```python
from build123d import *

# Parameters (mm, degrees)
F1_DEPTH = 63.5
F0_W     = 25.4
F0_H     = 19.05
F2_DEPTH = 25.4
F3_DEPTH = 15.875
F5_R     = 6.35


with BuildPart() as f1:
    # F0 (on Front) → F1 (new body, symmetric)
    with BuildSketch(Plane.XZ):
        Polygon((-41.275, 9.525), (-41.275, -9.525), (41.275, -9.525), (41.275, 9.525), (22.225, 9.525), align=None)
    extrude(amount=F1_DEPTH, both=True)

    # F0 (on Front) → F2 (join, symmetric)
    with BuildSketch(Plane.XZ):
        Polygon((60.325, 66.675), (60.325, 61.9252), (85.725, 61.9252), (85.725, 42.8752), (60.325, 42.8752), (60.325, 34.925), (111.125, 34.925), (111.125, 66.675), align=None)
        with BuildLine():
            Line((22.225, 9.525), (41.275, 9.525))
            Line((41.275, 9.525), (41.275, 27.0002))
            ThreePointArc((41.275, 27.0002), (45.92468, 38.22552), (57.15, 42.8752))
            Line((57.15, 42.8752), (60.325, 42.8752))
            Line((60.325, 42.8752), (60.325, 61.9252))
            Line((60.325, 61.9252), (57.15, 61.9252))
            ThreePointArc((57.15, 61.9252), (32.454296, 51.695904), (22.225, 27.0002))
            Line((22.225, 27.0002), (22.225, 9.525))
        make_face()
        with Locations((73.025, 52.4002)):
            Rectangle(F0_W, F0_H)
    extrude(amount=F2_DEPTH, both=True)

    # F0 (on Front) → F3 (join)
    with BuildSketch(Plane.XZ):
        with BuildLine():
            add(Edge.make_bspline(
                [(-41.275, 9.525), (-27.823856, 40.664345), (5.336885, 65.223247), (57.15, 61.9252)],
                knots=[0, 0, 0, 0, 111.504536, 111.504536, 111.504536, 111.504536], degree=3))
            Line((-41.275, 9.525), (22.225, 9.525))
            Line((22.225, 9.525), (22.225, 27.0002))
            ThreePointArc((22.225, 27.0002), (32.454296, 51.695904), (57.15, 61.9252))
        make_face()
    extrude(amount=F3_DEPTH)

    # F0 (on Front) → F4 (revolve)
    with BuildSketch(Plane.XZ):
        Polygon((60.325, 66.675), (60.325, 61.9252), (85.725, 61.9252), (85.725, 42.8752), (60.325, 42.8752), (60.325, 34.925), (111.125, 34.925), (111.125, 66.675), align=None)
    revolve(axis=Axis((111.125, 0, 50.8), (0, 0, 1)))

    # F5
    f5_edges = [f1.edges().sort_by_distance(p)[0] for p in [
        (-41.275, -63.5, 0),
        (41.275, -63.5, 0),
        (41.275, 63.5, 0),
        (-41.275, 63.5, 0),
    ]]
    fillet(f5_edges, radius=F5_R)


solid = f1.part
```
Can you work these out from the model? Positions are in its coordinate system, mm. A direction names the side the tool comes from. Coordinates: 2 decimals unless noted, no trailing zeros. Loops run counter-clockwise (first coordinate to the right, second up) from the corner with the lowest first, then second, coordinate; pieces in that order, holes last.
1) Imagine slicing it at A-A on y = 47. List the corners of the cut face in (x, z) for me (3 decimals), plus the area to 3 significant figures.
2) I need wall thicknesses on probe 1 along Z at (x, y) = (141, -13.5) (3 decimals); probe 2 along Z at (x, y) = (79, 10) (3 decimals); probe 3 along X at (y, z) = (-9, -2) (3 decimals). Which ranges of each line are inside material? Lowest first, please.
3) Which directions (+Z, -Z, +X, -X, +Y, -Y) give clear straight access to the entire face, cutting with the end or side of a thin tool? Please do faces 1 (the flat face through (-2, -15.875, 32)), 2 (the flat face through (135, 11, 42.875)), 3 (the cylindrical face through (45.8, -0.4, 38.1)).
4) Thinking about a two-plate mould opening in Z: for faces 4 (the cylindrical face through (32.73, 12.52, 51.97)), 5 (the flat face through (56, -25.4, 45)), 6 (the cylindrical face through (39.365, 61.689, 0.133)), 7 (the flat face through (136, 11, 61.925)), which applies, pulls with the +Z half, pulls with the -Z half, needs draft (parallel to the pull), parting line crosses it, or undercut?
5) For pin 1 (2.5 mm diameter, centred on x = 58.5, y = 5, fed in from +Z); pin 2 (1 mm diameter, centred on x = 69, z = 33.5, fed in from +Y); pin 3 (2.5 mm diameter, centred on y = -11, z = 38, fed in from -X); pin 4 (10 mm diameter, centred on x = 104.5, y = -28.5, fed in from -Z) (3 decimals), each with a flat end and sliding along its axis, tell me the tip position at first contact or that it passes through.
6) Imagine slicing it at B-B on z = 7. List the corners of the cut face in (x, y) for me (3 decimals).
7) Imagine slicing it at C-C on y = 5.5. List the corners of the cut face in (x, z) for me (3 decimals), plus the area to 3 significant figures.
8) Imagine slicing it at D-D on y = 30. List the corners of the cut face in (x, z) for me (3 decimals).
Completed:
1. outline: (-41.275, -9.525) - (41.275, -9.525) - (41.275, 9.525) - (-41.275, 9.525) - close; (91.847, 34.925) - (130.403, 34.925) - (130.403, 42.875) - (91.847, 42.875) - close; (91.847, 61.925) - (130.403, 61.925) - (130.403, 66.675) - (91.847, 66.675) - close
1. area: 2,060 mm2
2. probe 1: z = 34.925 to 42.875, 61.925 to 66.675
2. probe 2: z = 34.925 to 66.675
2. probe 3: x = -41.275 to 41.275
3. face 1: +Z, -X, -Y
3. face 2: +X
3. face 3: -Z, +Y, -Y
4. face 4: pulls with the +Z half
4. face 5: undercut
4. face 6: needs draft
4. face 7: undercut
5. pin 1: stops at z = 61.93
5. pin 2: passes through
5. pin 3: stops at x = -22.29
5. pin 4: stops at z = 34.925
6. outline: (-41.275, -57.15) arc R6.35 ccw to (-34.925, -63.5) - (34.925, -63.5) arc R6.35 ccw to (41.275, -57.15) - (41.275, 57.15) arc R6.35 ccw to (34.925, 63.5) - (-34.925, 63.5) arc R6.35 ccw to (-41.275, 57.15) - close
7. outline: (-41.275, -9.525) - (41.275, -9.525) - (41.275, 27) arc R15.875 cw to (57.15, 42.875) - (60.325, 42.875) - (60.325, 34.925) - (161.626, 34.925) - (161.626, 42.875) - (135.922, 42.875) - (135.922, 61.925) - (161.626, 61.925) - (161.626, 66.675) - (60.325, 66.675) - (60.325, 61.925) - (57.15, 61.925) arc R34.925 ccw to (22.225, 27) - (22.225, 9.525) - (-41.275, 9.525) - close
7. area: 5,450 mm2
8. outline: (-41.275, -9.525) - (41.275, -9.525) - (41.275, 9.525) - (-41.275, 9.525) - close; (70.129, 34.925) - (152.121, 34.925) - (152.121, 42.875) - (70.129, 42.875) - close; (70.129, 61.925) - (152.121, 61.925) - (152.121, 66.675) - (70.129, 66.675) - close
